Part model, mm, in its own coordinate system. Round coordinates to 2 decimals unless told otherwise and drop trailing zeros. Loops run counter-clockwise (first coordinate to the right, second up) from the corner with the lowest first, then second, coordinate; pieces in that order, holes last.
(1) Cut at A-A on x = 0. List the corners of the cut face in (y, z), then the cut area to 3 significant figures.
(2) Flat gauge pins, fed straight in: pin 1 (2.5 mm diameter, centred on x = 0, y = 0, fed in from -Z); pin 2 (4 mm diameter, centred on x = -1, y = 174.5, fed in from +Z); pin 3 (4 mm diameter, centred on x = 2, y = -21.5, fed in from +Z) (3 decimals). Where does each tip first touch, or does it go through?
(3) Cut at C-C on y = 223. List the corners of the cut face in (x, z) (3 decimals), then the cut area to 3 significant figures.
(4) Cut at B-B on z = 3.25. List the corners of the cut face in (x, y).
(5) Probe probe 1 along Y at (x, z) = (0, 0.35); probe 2 along X at (y, z) = (-348, 5); probe 3 along X at (y, z) = (0, 0.45). List the from-to ranges inside material, lowest first.
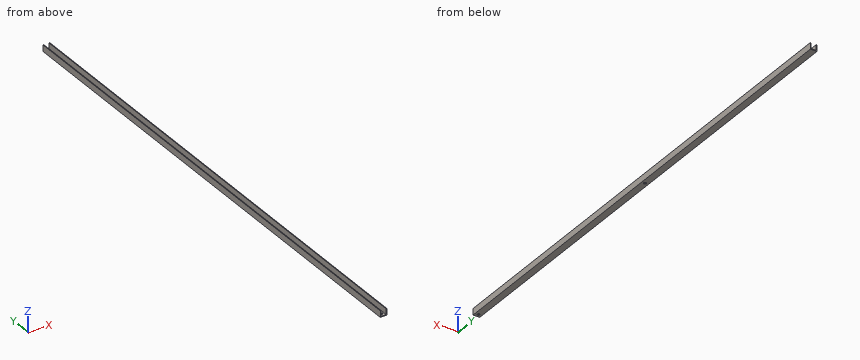
from build123d import *

# Parameters (mm, degrees)
F1_DEPTH      = 381
F1_DEPTH_BACK = 381
F2_R          = 2
F3_DEPTH      = 1.2
F4_R          = 2
F5_DEPTH      = 9.526


with BuildPart() as f1:
    # F0 (on Front) → F1 (new body, two sides)
    with BuildSketch(Plane.XZ) as f1_sk:
        Polygon((-3.8062, 9.525), (-5, 9.525), (-5, 0), (0, 0), (5, 0), (5, 9.525), (3.8062, 9.525), (3.8062, 1.2), (-3.8062, 1.2), align=None)
    extrude(amount=F1_DEPTH)
    extrude(f1_sk.sketch, amount=-F1_DEPTH_BACK)

    # F2 (on face) → F3 (cut, through all)
    with BuildSketch(Plane(origin=(0, 0, 0), x_dir=(1, 0, 0), z_dir=(0, 0, -1))):
        Circle(F2_R)
    extrude(amount=-F3_DEPTH, mode=Mode.SUBTRACT)

    # F4 (on face) → F5 (cut, through all)
    with BuildSketch(Plane(origin=(0, 0, 0), x_dir=(1, 0, 0), z_dir=(0, 0, -1))):
        with Locations((0, 376)):
            Circle(F4_R)
    extrude(amount=-F5_DEPTH, mode=Mode.SUBTRACT)


solid = f1.part
Final values:
1. outline: (-381, 0) - (-378, 0) - (-378, 1.2) - (-381, 1.2) - close; (-374, 0) - (-2, 0) - (-2, 1.2) - (-374, 1.2) - close; (2, 0) - (381, 0) - (381, 1.2) - (2, 1.2) - close
1. area: 905 mm2
2. pin 1: passes through
2. pin 2: stops at z = 1.2
2. pin 3: stops at z = 9.525
3. outline: (-5, 0) - (5, 0) - (5, 9.525) - (3.806, 9.525) - (3.806, 1.2) - (-3.806, 1.2) - (-3.806, 9.525) - (-5, 9.525) - close
3. area: 31.9 mm2
4. outline: (-5, -381) - (-3.81, -381) - (-3.81, 381) - (-5, 381) - close; (3.81, -381) - (5, -381) - (5, 381) - (3.81, 381) - close
5. probe 1: y = -381 to -378, -374 to -2, 2 to 381
5. probe 2: x = -5 to -3.81, 3.81 to 5
5. probe 3: x = -5 to -2, 2 to 5
